Design review of the part built by this model. Coordinates are the model's own, in mm. Face numbers are marked on the shaded views. A direction names the side the tool comes from. Coordinates: 2 decimals unless noted, no trailing zeros. Loops run counter-clockwise (first coordinate to the right, second up) from the corner with the lowest first, then second, coordinate; pieces in that order, holes last.
Q1. Add section C-C on x = -13. Give the boundary of the cut face in (y, z).
Q2. Add section D-D on y = 0. Give the boundary of the cut face in (x, z).
Q3. Add section B-B on y = 7. Give the boundary of the cut face in (x, z), and give its area (3 significant figures).
Q4. Wall thickness on probe 1 along Z at (x, y) = (-2.5, 4.5); probe 2 along Z at (x, y) = (9.5, -15); probe 3 along Y at (x, z) = (10.5, -10): over which ranges is each line inside the solid? List them lowest first.
Q5. Add section A-A on z = 30. Give the boundary of the cut face in (x, y).
Q6. For P1, Ø8, axis at x = -17, y = 7, coming from the -Z side; P2, Ø8, axis at x = -6.5, y = -11.5, coming from the -Z side; P3, Ø0.8, axis at x = -0.5, y = 3.5, coming from the -Z side, all flat-tipped, find the tip position at first contact; note any pin that passes through.
Q7. Machinability: for the marked faces 1 and 2, which of the approach directions +Z, -Z, +X, -X, +Y, -Y give a long, thin tool a straight path to every point of the face, cutting with its end or side? Answer none if there is none.
```python
from build123d import *

# Parameters (mm, degrees)
SKETCH_W     = 42
SKETCH_H     = 42
PAD_DEPTH    = 40
CHAMFER_SIZE = 4
SKETCH005_R  = 18
PAD003_DEPTH = 27.3
SKETCH001_R  = 11
PAD001_DEPTH = 2
SKETCH002_R  = 4
PAD002_DEPTH = 20
POCKET_DEPTH = 15
SKETCH004_R  = 1.25
HOLE_DEPTH   = 4.5
HOLE_TIPS_R  = 1.25


with BuildPart() as part:
    # Sketch → Pad (new body)
    with BuildSketch(Plane.XY):
        Rectangle(SKETCH_W, SKETCH_H)
    extrude(amount=PAD_DEPTH)

    # Chamfer
    chamfer_edges = [part.edges().sort_by_distance(p)[0] for p in [
        (21, -21, 20),
        (-21, -21, 20),
        (21, 21, 20),
        (-21, 21, 20),
    ]]
    chamfer(chamfer_edges, length=CHAMFER_SIZE)

    # Sketch005 → Pad003 (join)
    with BuildSketch(Plane.XY):
        Circle(SKETCH005_R)
    extrude(amount=-PAD003_DEPTH)

    # Sketch001 → Pad001 (join)
    with BuildSketch(Plane.XY.offset(-27.3)):
        Circle(SKETCH001_R)
    extrude(amount=-PAD001_DEPTH)

    # Sketch002 (on Sketch) → Pad002 (join)
    with BuildSketch(Plane.XY.offset(-27.3)):
        Circle(SKETCH002_R)
    extrude(amount=-PAD002_DEPTH)

    # Sketch003 (on Sketch) → Pocket (cut)
    with BuildSketch(Plane.XY.offset(-32.3)):
        with BuildLine():
            ThreePointArc((10.583005, 3), (0, 11), (-10.583005, 3))
            Line((-10.583005, 3), (10.583005, 3))
        make_face()
    extrude(amount=-POCKET_DEPTH, mode=Mode.SUBTRACT)

    # Sketch004 (on Sketch) → Hole (cut)
    with BuildSketch(Plane.XY.offset(-27.3)):
        with Locations((9.899495, 9.899495)):
            Circle(SKETCH004_R)
        with Locations((-9.899495, 9.899495)):
            Circle(SKETCH004_R)
        with Locations((-9.899495, -9.899495)):
            Circle(SKETCH004_R)
        with Locations((9.899495, -9.899495)):
            Circle(SKETCH004_R)
    extrude(amount=HOLE_DEPTH, mode=Mode.SUBTRACT)

    # Hole tips → Hole tip 1 section 0
    with BuildSketch(Plane.XY.offset(-22.8), mode=Mode.PRIVATE) as hole_tip_1_s0:
        with Locations((9.899495, 9.899495)):
            Circle(HOLE_TIPS_R)
    loft([hole_tip_1_s0.sketch, Vertex(9.899495, 9.899495, -22.048924)], mode=Mode.SUBTRACT)

    # Hole tips → Hole tip 2 section 0
    with BuildSketch(Plane.XY.offset(-22.8), mode=Mode.PRIVATE) as hole_tip_2_s0:
        with Locations((-9.899495, 9.899495)):
            Circle(HOLE_TIPS_R)
    loft([hole_tip_2_s0.sketch, Vertex(-9.899495, 9.899495, -22.048924)], mode=Mode.SUBTRACT)

    # Hole tips → Hole tip 3 section 0
    with BuildSketch(Plane.XY.offset(-22.8), mode=Mode.PRIVATE) as hole_tip_3_s0:
        with Locations((-9.899495, -9.899495)):
            Circle(HOLE_TIPS_R)
    loft([hole_tip_3_s0.sketch, Vertex(-9.899495, -9.899495, -22.048924)], mode=Mode.SUBTRACT)

    # Hole tips → Hole tip 4 section 0
    with BuildSketch(Plane.XY.offset(-22.8), mode=Mode.PRIVATE) as hole_tip_4_s0:
        with Locations((9.899495, -9.899495)):
            Circle(HOLE_TIPS_R)
    loft([hole_tip_4_s0.sketch, Vertex(9.899495, -9.899495, -22.048924)], mode=Mode.SUBTRACT)


solid = part.part
```
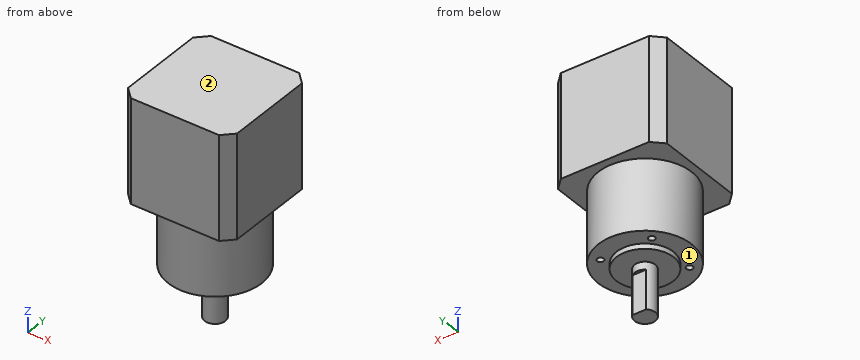
Entries:
1. outline: (-21, 0) - (-12.45, 0) - (-12.45, -27.3) - (12.45, -27.3) - (12.45, 0) - (21, 0) - (21, 40) - (-21, 40) - close
2. outline: (-21, 0) - (-18, 0) - (-18, -27.3) - (-11, -27.3) - (-11, -29.3) - (-4, -29.3) - (-4, -47.3) - (4, -47.3) - (4, -29.3) - (11, -29.3) - (11, -27.3) - (18, -27.3) - (18, 0) - (21, 0) - (21, 40) - (-21, 40) - close
3. outline: (-21, 0) - (-16.58, 0) - (-16.58, -27.3) - (-8.49, -27.3) - (-8.49, -29.3) - (8.49, -29.3) - (8.49, -27.3) - (16.58, -27.3) - (16.58, 0) - (21, 0) - (21, 40) - (-21, 40) - close
3. area: 2,620 mm2
4. probe 1: z = -29.3 to 40
4. probe 2: z = -27.3 to 40
4. probe 3: y = -14.62 to 14.62
5. outline: (-21, -17) - (-17, -21) - (17, -21) - (21, -17) - (21, 17) - (17, 21) - (-17, 21) - (-21, 17) - close
6. P1: stops at z = -27.3
6. P2: stops at z = -29.3
6. P3: stops at z = -32.3
7. face 1: -Z
7. face 2: +Z, +X, -X, +Y, -Y
